Can you work these out from the model? Positions are in its coordinate system, mm. A direction names the side the tool comes from. Coordinates: 2 decimals unless noted, no trailing zeros. Order: outer loops, then holes, each group sorted by start corner. A loop starts at its lowest first (then second) coordinate and runs counter-clockwise, first axis right, second up.
```python
from build123d import *

# Parameters (mm, degrees)
SKETCH_1_W               = 60
SKETCH_1_H               = 48
EXTRUDE_1_DEPTH          = 8
SKETCH_3_W               = 65
SKETCH_3_H               = 15
EXTRUDE_2_DEPTH          = 8
SKETCH_5_R               = 1.8
CUT_EXTRUDE_1_DEPTH      = 3
MIRROR_3_COPY_1_SKETCH_R = 1.8
MIRROR_3_COPY_1_DEPTH    = 3
SKETCH_7_R               = 10
CUT_EXTRUDE_2_DEPTH      = 8


with BuildPart() as part:
    # Sketch 1 → Extrude 1 (new body)
    with BuildSketch(Plane.XY):
        Rectangle(SKETCH_1_W, SKETCH_1_H)
    extrude(amount=EXTRUDE_1_DEPTH)

    # Sketch 3 → Extrude 2 (add)
    with BuildSketch(Plane.XY.offset(8)):
        Rectangle(SKETCH_3_W, SKETCH_3_H)
    extrude(amount=-EXTRUDE_2_DEPTH)

    # Sketch 5 → Cut-Extrude 1 (cut)
    with BuildSketch(Plane(origin=(30, 0, 0), x_dir=(0, 0, -1), z_dir=(1, 0, 0))):
        with Locations((-4, 21)):
            Circle(SKETCH_5_R)
    cut_extrude_1 = extrude(amount=-CUT_EXTRUDE_1_DEPTH, mode=Mode.SUBTRACT)

    # Mirror 2: Cut-Extrude 1 across plane
    add(cut_extrude_1.mirror(Plane.ZX), mode=Mode.SUBTRACT)

    # Mirror 3: Cut-Extrude 1 across plane
    add(cut_extrude_1.mirror(Plane(origin=(0, 0, 0), x_dir=(0, 0, 1), z_dir=(1, 0, 0))), mode=Mode.SUBTRACT)

    # Mirror 3 copy 1 sketch → Mirror 3 copy 1 (cut)
    with BuildSketch(Plane(origin=(-30, 0, 0), x_dir=(0, 0, -1), z_dir=(-1, 0, 0))):
        with Locations((-4, 21)):
            Circle(MIRROR_3_COPY_1_SKETCH_R)
    extrude(amount=-MIRROR_3_COPY_1_DEPTH, mode=Mode.SUBTRACT)

    # Sketch 7 → Cut-Extrude 2 (cut)
    with BuildSketch(Plane.XY.offset(8)):
        Circle(SKETCH_7_R)
    extrude(amount=-CUT_EXTRUDE_2_DEPTH, mode=Mode.SUBTRACT)


solid = part.part
```
1. Imagine slicing it at D-D on y = 21. Please give me the cut outline in (x, z), then the cut area to 3 significant figures.
Completed:
outline: (-30, 0) - (30, 0) - (30, 2.2) - (27, 2.2) - (27, 5.8) - (30, 5.8) - (30, 8) - (-30, 8) - (-30, 5.8) - (-27, 5.8) - (-27, 2.2) - (-30, 2.2) - close
area: 458 mm2
2. Imagine slicing it at C-C on y = 0. Please give me the cut outline in (x, z).
Completed:
outline: (-32.5, 0) - (-10, 0) - (-10, 8) - (-32.5, 8) - close; (10, 0) - (32.5, 0) - (32.5, 8) - (10, 8) - close
3. On a 3-axis mill with a long thin cutter (end or side, diameter ignored), from which of +Z, -Z, +X, -X, +Y, -Y can I reach the whole of each face in a straight line? I mean faces 4 (the flat face through (-30, 16, 4)), 5 (the flat face through (-31, -7.5, 4)), 6 (the cylindrical face through (28.521, 22.518, 3.032)). Say none if no direction works.
Completed:
face 4: +Z, -Z, -X, +Y
face 5: +Z, -Z, -X, -Y
face 6: +X
4. Please list where these lines run through material, in increasing order: probe 1 along Y at (x, z) = (28.1, 4); probe 2 along Y at (x, z) = (0, 4.5); probe 3 along X at (y, z) = (-13, 6.5).
Completed:
probe 1: y = -24 to -22.8, -19.2 to 19.2, 22.8 to 24
probe 2: y = -24 to -10, 10 to 24
probe 3: x = -30 to 30
5. Imagine slicing it at A-A on x = 0. Please give me the cut outline in (y, z), then the cut area to 3 significant figures.
Completed:
outline: (-24, 0) - (-10, 0) - (-10, 8) - (-24, 8) - close; (10, 0) - (24, 0) - (24, 8) - (10, 8) - close
area: 224 mm2
6. I'm going to push flat-ended pins straight in: pin 1 (4.5 mm diameter, centred on y = 21, z = 4, fed in from -X); pin 2 (0.8 mm diameter, centred on x = -31.5, z = 4, fed in from -Y); pin 3 (3 mm diameter, centred on y = -21, z = 4, fed in from +X); pin 4 (8 mm diameter, centred on x = 13.5, y = 12.5, fed in from -Z). Where does each tip first touch, or does it pass through?
Completed:
pin 1: stops at x = -30
pin 2: stops at y = -7.5
pin 3: stops at x = 27
pin 4: stops at z = 0
7. Imagine slicing it at B-B on z = 6.5. Please give me the cut outline in (x, y), then the cut area to 3 significant figures.
Completed:
outline: (-32.5, -7.5) - (-30, -7.5) - (-30, -24) - (30, -24) - (30, -7.5) - (32.5, -7.5) - (32.5, 7.5) - (30, 7.5) - (30, 24) - (-30, 24) - (-30, 7.5) - (-32.5, 7.5) - close; hole circle Ø20 at (0, 0)
area: 2,640 mm2
8. Thinking about a two-plate mould opening in Z: for faces 1 (the flat face through (0, 11, 0)), 2 (the flat face through (-27, 21, 4)), 3 (the flat face through (-30, -16, 4)), which applies, pulls with the +Z half, pulls with the -Z half, needs draft (parallel to the pull), parting line crosses it, or undercut?
Completed:
face 1: pulls with the -Z half
face 2: undercut
face 3: needs draft
